from build123d import *

# Parameters (mm, degrees)
SKETCH1_R           = 66.5
SKETCH1_R_2         = 3.75
SKETCH1_R_3         = 0.875
BOSS_EXTRUDE1_DEPTH = 4
BOSS_EXTRUDE2_DEPTH = 25
CUT_EXTRUDE1_DEPTH  = 11
CUT_EXTRUDE2_DEPTH  = 12
SKETCH6_3_R         = 0.875
CUT_EXTRUDE3_DEPTH  = 8
SKETCH7_R           = 10.5
CUT_EXTRUDE4_DEPTH  = 122.239616981
SKETCH8_W           = 7.5
SKETCH8_H           = 10
BOSS_EXTRUDE3_DEPTH = 8
SKETCH9_W           = 6
SKETCH9_H           = 4
CUT_EXTRUDE5_DEPTH  = 8
CUT_EXTRUDE6_REACH  = 114.543
SKETCH10_W          = 7.5
SKETCH10_H          = 2


with BuildPart() as part:
    # Sketch1 → Boss-Extrude1 (new body)
    with BuildSketch(Plane(origin=(0, 0, 0), x_dir=(1, 0, 0), z_dir=(0, 1, 0))):
        with Locations(Location((0, 0, 0), (0, 0, 270))):
            Circle(SKETCH1_R)
        with Locations(Location((0, 0, 0), (0, 0, 270))):
            Circle(SKETCH1_R_2, mode=Mode.SUBTRACT)
        with Locations(Location((0, -7.25, 0), (0, 0, 270))):
            Circle(SKETCH1_R_3, mode=Mode.SUBTRACT)
        with Locations(Location((0, 7.25, 0), (0, 0, 270))):
            Circle(SKETCH1_R_3, mode=Mode.SUBTRACT)
    extrude(amount=-BOSS_EXTRUDE1_DEPTH)

    # Sketch4 → Boss-Extrude2 (add)
    with BuildSketch(Plane(origin=(5, 0, 0), x_dir=(0, 0, -1), z_dir=(1, 0, 0))):
        with BuildLine():
            Line((0, 0), (35, 0))
            Line((35, 0), (7.77909307, 58.375423293))
            ThreePointArc((7.77909307, 58.375423293), (-14.471447396, 69.348175551), (-30, 50))
            Line((-30, 50), (-30, 0))
            Line((-30, 0), (0, 0))
        make_face()
    extrude(amount=BOSS_EXTRUDE2_DEPTH)

    # Sketch5 → Cut-Extrude1 (cut)
    with BuildSketch(Plane(origin=(30, 0, 0), x_dir=(0, 0, -1), z_dir=(1, 0, 0))):
        with BuildLine():
            Line((-27, 3), (-27, 0))
            Line((-27, 0), (30.290943269, 0))
            Line((30.290943269, 0), (30.290943269, 3))
            Line((30.290943269, 3), (5.060169709, 57.107568508))
            ThreePointArc((5.060169709, 57.107568508), (-13.822128554, 66.419287529), (-27, 50))
            Line((-27, 50), (-27, 3))
        make_face()
    extrude(amount=-CUT_EXTRUDE1_DEPTH, mode=Mode.SUBTRACT)

    # Sketch6 → Cut-Extrude2 (cut)
    with BuildSketch(Plane(origin=(19, 0, 0), x_dir=(0, 0, -1), z_dir=(1, 0, 0))):
        Polygon((-16.515307171, 49.483019708), (-21.5, 47.158619269), (-4.172651269, 10), (0.81204156, 12.32440044), align=None)
        Polygon((-7.452229301, 53.709202325), (-16.515307171, 49.483019708), (0.81204156, 12.32440044), (9.87511943, 16.550583057), align=None)
        Polygon((-2.467536472, 56.033602765), (-7.452229301, 53.709202325), (9.87511943, 16.550583057), (14.859812259, 18.874983497), align=None)
    extrude(amount=-CUT_EXTRUDE2_DEPTH, mode=Mode.SUBTRACT)

    # Sketch6_3 → Cut-Extrude3 (cut)
    with BuildSketch(Plane(origin=(19, 0, 0), x_dir=(0, 0, -1), z_dir=(1, 0, 0))):
        with Locations((-17.994471087, 52.655096963)):
            Circle(SKETCH6_3_R)
        with Locations((-8.931393217, 56.88127958)):
            Circle(SKETCH6_3_R)
        with Locations((11.354283347, 13.378505802)):
            Circle(SKETCH6_3_R)
        with Locations((2.291205476, 9.152323185)):
            Circle(SKETCH6_3_R)
    extrude(amount=-CUT_EXTRUDE3_DEPTH, mode=Mode.SUBTRACT)

    # Sketch7 → Cut-Extrude4 (cut, through all)
    with BuildSketch(Plane(origin=(7, 0, 0), x_dir=(0, 0, -1), z_dir=(1, 0, 0))):
        with Locations(Location((-7.546276488, 42.079879253, 0), (0, 0, 25))):
            Circle(SKETCH7_R)
    extrude(amount=-CUT_EXTRUDE4_DEPTH, mode=Mode.SUBTRACT)

    # Sketch8 → Boss-Extrude3 (add)
    with BuildSketch(Plane(origin=(0, 0, 0), x_dir=(1, 0, 0), z_dir=(0, 1, 0))):
        with Locations((-3.75, 32)):
            Rectangle(SKETCH8_W, SKETCH8_H)
    extrude(amount=BOSS_EXTRUDE3_DEPTH)

    # Sketch9 → Cut-Extrude5 (cut)
    with BuildSketch(Plane.ZY.offset(7.5)):
        with Locations((-32, 4)):
            Rectangle(SKETCH9_W, SKETCH9_H)
    extrude(amount=-CUT_EXTRUDE5_DEPTH, mode=Mode.SUBTRACT)

    # Sketch10 → Cut-Extrude6 (cut, up to next)
    with BuildSketch(Plane(origin=(0, 8, 0), x_dir=(1, 0, 0), z_dir=(0, 1, 0)), mode=Mode.PRIVATE) as cut_extrude6_sk1:
        with Locations((-3.75, 34)):
            Rectangle(SKETCH10_W, SKETCH10_H)
    cut_extrude6_tool1 = extrude(cut_extrude6_sk1.sketch, amount=-CUT_EXTRUDE6_REACH, mode=Mode.PRIVATE) & part.part
    add(cut_extrude6_tool1.solids().sort_by_distance((-3.75, 8, -34))[0], mode=Mode.SUBTRACT)


solid = part.part
CAD build for the part. Positions are in the model's coordinates, mm. A direction names the side the tool comes from. Round coordinates to 2 decimals unless told otherwise and drop trailing zeros. Write each loop counter-clockwise with the first axis right and the second up, starting at its lowest first coordinate (ties: lowest second). Pieces come first, ordered by that corner, then holes. Notation, with made-up numbers: M -23.75,61.5 L 22.25,61.5 A25 cw 22.25,84.5 Z; hole C 6,31.25 d2. An arc over 180 degrees is marked long. Use a Markdown table: item, result. Add a question column.
1. 3-axis set-ups, long thin cutter, end or side, ignore diameter. For faces 1 (the face through (-4, 8, -30)), 2 (the face through (0, 1, -32)), 3 (the face through (-4, 4, -27)), 4 (the face through (-4, 2, -32)), 5 (the face through (13.08, 37.19, -6.32)): which of +Z, -Z, +X, -X, +Y, -Y reach the whole face in a straight line?
2. Flat gauge pins, fed straight in: P1, Ø9, axis at y = 2, z = -31.5, coming from the -X side; P2, Ø6.5, axis at x = -2.5, z = -32.5, coming from the +Y side; P3, Ø5, axis at y = 36, z = -14, coming from the +X side. Where does each tip first touch, or does it go through?
3. Slice it at A-A on y = 36. Give the cut face in (x, z), then the cut area to 3 significant figures.
4. Slice it at B-B on z = 25. Give the cut face in (x, y).
5. Pull direction Z, two halves, no side cores. Call faces 6 (the face through (17.325, 69.426, 14.104)), 7 (the face through (30, 43, -12)), 8 (the face through (0.165, -1.972, -3.746)): released by +Z, released by -Z, zero draft, split by the parting line, or undercut.
6. Drill centre lines: probe 1 along Y at (x, z) = (-1, -54); probe 2 along Z at (x, y) = (11, 54.5); probe 3 along X at (y, z) = (26.5, -7.5). Where is each one in solid material? Low to high.
7. Slice it at C-C on z = -58. Give the cut face in (x, y).
Reply:
| question | item | result |
|---|---|---|
| 1 | face 1 | +Z, -Z, -X, +Y |
| 1 | face 2 | +Z, -Z, +Y |
| 1 | face 3 | +Z, -X, +Y |
| 1 | face 4 | -X |
| 1 | face 5 | +X |
| 2 | P1 | stops at x = -60.56 |
| 2 | P2 | stops at y = 8 |
| 2 | P3 | stops at x = 30 |
| 3 | outline | M 5,-18.21 L 30,-18.21 L 30,-14.9 L 19,-14.9 L 19,-6.87 L 7,-6.87 L 7,-1.01 L 5,-1.01 Z; M 5,16.11 L 7,16.11 L 7,16.3 L 19,16.3 L 19,27 L 30,27 L 30,30 L 5,30 Z |
| 3 | area | 432 mm^2 |
| 4 | outline | M -61.62,-4 L 61.62,-4 L 61.62,0 L 19,0 L 19,57.95 L 30,57.95 L 30,63.16 L 5,63.16 L 5,0 L -61.62,0 Z |
| 5 | face 6 | split by the parting line |
| 5 | face 7 | zero draft |
| 5 | face 8 | undercut |
| 6 | probe 1 | y = -4 to 0 |
| 6 | probe 2 | z = -9.59 to 1.75, 5.76 to 29.48 |
| 6 | probe 3 | x = 5 to 7 |
| 7 | outline | M -32.53,-4 L 32.53,-4 L 32.53,0 L -32.53,0 Z |
